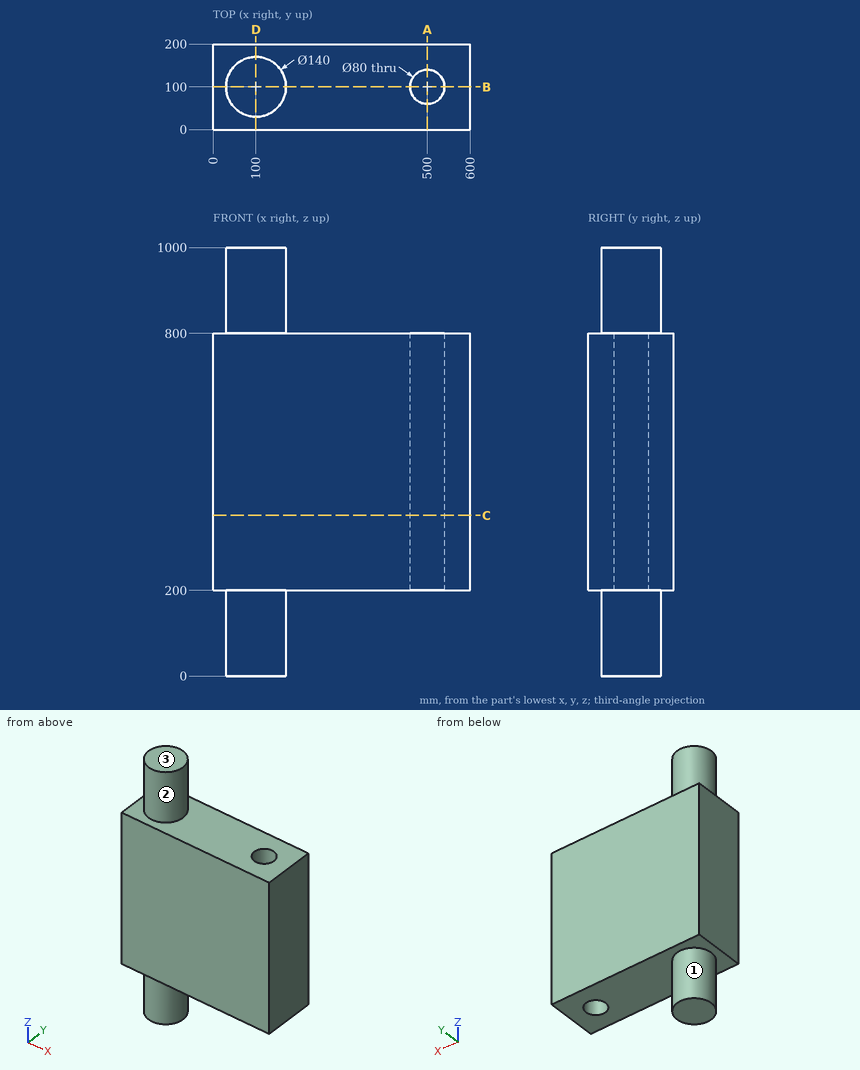
Can you work these out from the drawing? Everything is in mm from the part's minimum corner. A direction names the side the tool comes from. Round coordinates to 2 decimals unless told otherwise and drop trailing zeros. Order: outer loops, then holes, each group sorted by start corner. A loop starts at its lowest first (then second) coordinate and runs counter-clockwise, first axis right, second up.
(1) On a 3-axis mill with a long thin cutter (end or side, diameter ignored), from which of +Z, -Z, +X, -X, +Y, -Y can I reach the whole of each face in a straight line? I mean the marked faces 1, 2 and 3. Say none if no direction works.
Results are:
face 1: -Z
face 2: +Z
face 3: +Z, +X, -X, +Y, -Y
(2) If we section it at C-C (z = 375): Please give me the cut outline in (x, y), plus the area to 3 significant figures.
Results are:
outline: (0, 0) - (600, 0) - (600, 200) - (0, 200) - close; hole circle Ø80 at (500, 100)
area: 115,000 mm2
(3) If we section it at A-A (x = 500): Please give me the cut outline in (y, z).
Results are:
outline: (0, 200) - (60, 200) - (60, 800) - (0, 800) - close; (140, 200) - (200, 200) - (200, 800) - (140, 800) - close
(4) I'm going to push flat-ended pins straight in: pin 1 (10 mm diameter, centred on x = 416.5, y = 74, fed in from +Z); pin 2 (1.5 mm diameter, centred on x = 316, y = 46, fed in from -Z). Where does each tip first touch, or does it pass through?
Results are:
pin 1: stops at z = 800
pin 2: stops at z = 200
(5) If I drill on L1, parallel to X at y = 100, z = 484; L2, parallel to Y at x = 500, z = 651.5; L3, parallel to Z at x = 169, y = 173, over which ranges is the centre line in solid material (lowest first)?
Results are:
L1: x = 0 to 460, 540 to 600
L2: y = 0 to 60, 140 to 200
L3: z = 200 to 800
(6) If we section it at D-D (x = 100): Please give me the cut outline in (y, z).
Results are:
outline: (0, 200) - (30, 200) - (30, 0) - (170, 0) - (170, 200) - (200, 200) - (200, 800) - (170, 800) - (170, 1000) - (30, 1000) - (30, 800) - (0, 800) - close
(7) If we section it at B-B (y = 100): Please give me the cut outline in (x, z), plus the area to 3 significant figures.
Results are:
outline: (0, 200) - (30, 200) - (30, 0) - (170, 0) - (170, 200) - (460, 200) - (460, 800) - (170, 800) - (170, 1000) - (30, 1000) - (30, 800) - (0, 800) - close; (540, 200) - (600, 200) - (600, 800) - (540, 800) - close
area: 368,000 mm2
